from build123d import *

# Parameters (mm, degrees)
F0_W      = 8
F0_H      = 8
F1_DEPTH  = 8
F2_DEPTH  = 16
F4_DEPTH  = 8
F5_DEPTH  = 16
F0_W_2    = 16
F0_H_2    = 16
F6_DEPTH  = 8
F7_W      = 8
F7_H      = 16
F8_DEPTH  = 8
F10_DEPTH = 8


with BuildPart() as f1:
    # F0 (on Front) → F1 (new body)
    with BuildSketch(Plane.XZ):
        with Locations((-40.0961564034, 37.5077876064)):
            Rectangle(F0_W, F0_H)
    extrude(amount=F1_DEPTH)

    # F0 (on Front) → F2 (join)
    with BuildSketch(Plane.XZ):
        Polygon((-44.0961564034, 41.5077876064), (-60.0961564034, 41.5077876064), (-60.0961564034, 25.5077876064), (-44.0961564034, 25.5077876064), (-44.0961564034, 33.5077876064), align=None)
    extrude(amount=F2_DEPTH)

    # F3 (on face) → F4 (cut)
    with BuildSketch(Plane.YZ.offset(-36.0961564034)):
        Polygon((0, 33.5077876064), (-8, 41.5077876064), (-8, 33.5077876064), align=None)
    extrude(amount=-F4_DEPTH, mode=Mode.SUBTRACT)

    # F0 (on Front) → F5 (join)
    with BuildSketch(Plane.XZ):
        with Locations((-32.0961564034, 37.5077876064)):
            Rectangle(F0_W, F0_H)
    extrude(amount=F5_DEPTH)

    # F0 (on Front) → F6 (join)
    with BuildSketch(Plane.XZ):
        with Locations((-52.0961564034, 17.5077876064)):
            Rectangle(F0_W_2, F0_H_2)
    extrude(amount=F6_DEPTH)

    # F7 (on face) → F8 (join)
    with BuildSketch(Plane.XZ.offset(8)):
        with Locations((-48.0961564034, 17.5077876064)):
            Rectangle(F7_W, F7_H)
    extrude(amount=F8_DEPTH)

    # F9 (on face) → F10 (cut)
    with BuildSketch(Plane(origin=(-52.0961564034, 0, 0), x_dir=(0, -1, 0), z_dir=(-1, 0, 0))):
        Polygon((8, 25.5077876064), (16, 17.5077876064), (16, 25.5077876064), align=None)
    extrude(amount=-F10_DEPTH, mode=Mode.SUBTRACT)


solid = f1.part
The model under review builds one solid part; all positions refer to its coordinate system, in mm. A direction names the side the tool comes from. Round coordinates to 2 decimals unless told otherwise and drop trailing zeros. Loops run counter-clockwise (first coordinate to the right, second up) from the corner with the lowest first, then second, coordinate; pieces in that order, holes last. Notation, with made-up numbers: (3, -29) -> (26, -29) arc R38 cw to (26, 10) -> close; hole circle Ø2 at (1.5, -27.5). An arc over 180 degrees is marked (long way). Return JSON: item names as keys, results as strings.
(1) For faces 1 (the flat face through (-52.096, -12, 16)), 2 (the flat face through (-36.096, -10, 37)), 3 (the flat face through (-32, -8, 33.508)), 4 (the flat face through (-48.152, -11.944, 21.564)), list the 3-axis set-ups (+Z, -Z, +X, -X, +Y, -Y) from which the entire face can be reached by the end or side of a thin tool; tool diameter is ignored.
Solved:
{"face 1": "-Z, -X, -Y", "face 2": "-Z, -Y", "face 3": "-Z, +X, +Y, -Y", "face 4": "+X, -X, -Y"}
(2) Add section C-C on z = 38. Write out the cut boundary in (x, y), plus the area to 3 significant figures.
Solved:
{"outline": "(-60.1, -16) -> (-44.1, -16) -> (-44.1, -4.49) -> (-36.1, -4.49) -> (-36.1, -16) -> (-28.1, -16) -> (-28.1, 0) -> (-60.1, 0) -> close", "area": "420 mm2"}
(3) For line 1 (X direction, y = -10.75, z = 39); line 2 (X direction, y = -10.25, z = 27); line 3 (Z direction, x = -30.5, y = -12.25), list the stretches that pass through material, from the lowest coordinate up.
Solved:
{"line 1": "-60.1 to -44.1, -36.1 to -28.1", "line 2": "-60.1 to -44.1", "line 3": "33.51 to 41.51"}
(4) For pin 1 (9 mm diameter, centred on x = -57.5, z = 16, fed in from -Y); pin 2 (4 mm diameter, centred on x = -34, y = -4.5, fed in from -Z); pin 3 (2.5 mm diameter, centred on y = -10.5, z = 18.5, fed in from -X), all flat-tipped, find the tip position at first contact; note any pin that passes through.
Solved:
{"pin 1": "y = -8", "pin 2": "z = 33.51", "pin 3": "x = -52.1"}
(5) The part is to be moulded in two halves that separate along Z. For faces 5 (the flat face through (-44.3, -7.9, 41.508)), 6 (the flat face through (-40.04, -3.94, 37.45)), 7 (the flat face through (-52, -16, 34)), 8 (the flat face through (-52, -12, 25.508)), say which applies: released by +Z, released by -Z, zero draft, split by the parting line, or undercut.
Solved:
{"face 5": "released by +Z", "face 6": "released by -Z", "face 7": "zero draft", "face 8": "undercut"}
(6) Add section A-A on x = -46. Write out the cut boundary in (y, z), plus the area to 3 significant figures.
Solved:
{"outline": "(-16, 9.51) -> (0, 9.51) -> (0, 41.51) -> (-16, 41.51) -> (-16, 25.51) -> (-8, 25.51) -> (-16, 17.51) -> close", "area": "480 mm2"}
(7) Add section D-D on y = -1.25. Write out the cut boundary in (x, z).
Solved:
{"outline": "(-60.1, 9.51) -> (-44.1, 9.51) -> (-44.1, 34.76) -> (-36.1, 34.76) -> (-36.1, 33.51) -> (-28.1, 33.51) -> (-28.1, 41.51) -> (-60.1, 41.51) -> close"}
(8) Add section B-B on y = -13. Write out the cut boundary in (x, z), plus the area to 3 significant figures.
Solved:
{"outline": "(-60.1, 25.51) -> (-44.1, 25.51) -> (-44.1, 41.51) -> (-60.1, 41.51) -> close; (-52.1, 9.51) -> (-44.1, 9.51) -> (-44.1, 20.51) -> (-52.1, 20.51) -> close; (-36.1, 33.51) -> (-28.1, 33.51) -> (-28.1, 41.51) -> (-36.1, 41.51) -> close", "area": "408 mm2"}
